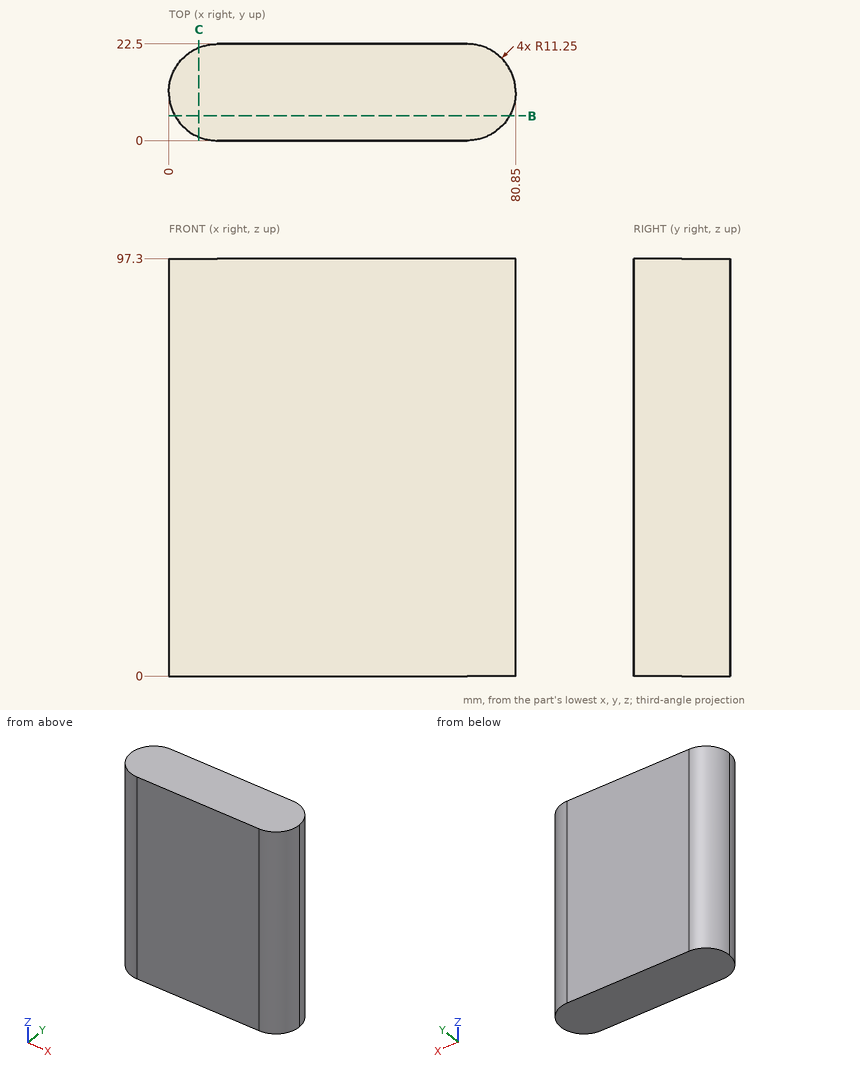
Drawing for the job (mm, zero at the part's lowest x, y, z). Round coordinates to 2 decimals unless told otherwise and drop trailing zeros. Order: outer loops, then holes, each group sorted by start corner. A loop starts at its lowest first (then second) coordinate and runs counter-clockwise, first axis right, second up.
Item 1: Probe line 1 along Y through (x, z) = (10, 36); line 2 along X through (y, z) = (9, 50); line 3 along X through (y, z) = (5, 63). List the from-to ranges inside material, lowest first.
Item 2: Pin check, flat tips, straight feed: pin 1 (12 mm diameter, centred on y = 4, z = 78.5, fed in from +X); pin 2 (1.5 mm diameter, centred on y = 18.5, z = 10, fed in from +X); pin 3 (1 mm diameter, centred on y = 15.5, z = 42.5, fed in from +X). Stop position of each tip, or through.
Item 3: Saw through at B-B on y = 5.75. Write the cut outline in (x, z), then the cut area to 3 significant figures.
Item 4: Saw through at C-C on x = 7. Write the cut outline in (y, z).
Reported:
1. line 1: y = 0.07 to 22.43
1. line 2: x = 0.23 to 80.62
1. line 3: x = 1.9 to 78.95
2. pin 1: stops at x = 80.78
2. pin 2: stops at x = 78.78
2. pin 3: stops at x = 80.21
3. outline: (1.44, 0) - (79.41, 0) - (79.41, 97.3) - (1.44, 97.3) - close
3. area: 7,590 mm2
4. outline: (0.83, 0) - (21.67, 0) - (21.67, 97.3) - (0.83, 97.3) - close
